```python
from build123d import *

# Parameters (mm, degrees)
SCHIZZO2_R                   = 25.5
TAGLIO_ESTRUSIONE1_DEPTH     = 10
ESTRUSIONE_ESTRUSIONE1_DEPTH = 51
TAGLIO_ESTRUSIONE2_DEPTH     = 51
SCHIZZO6_R                   = 38.5
TAGLIO_ESTRUSIONE3_DEPTH     = 51


with BuildPart() as part:
    # Schizzo1 → Rivoluzione1 (revolve)
    with BuildSketch(Plane.XY):
        Polygon((0, 439), (101.5, 439), (101.5, 0), (76, 0), (76, 413.5), (0, 413.5), align=None)
    revolve(axis=Axis((0, -167.269578169, 0), (0, 1, 0)))

    # Schizzo2 → Taglio-Estrusione1 (cut)
    with BuildSketch(Plane(origin=(0, 439, 0), x_dir=(1, 0, 0), z_dir=(0, 1, 0))):
        Circle(SCHIZZO2_R)
    extrude(amount=-TAGLIO_ESTRUSIONE1_DEPTH, mode=Mode.SUBTRACT)

    # Schizzo4 → Estrusione-Estrusione1 (add)
    with BuildSketch(Plane(origin=(190.786805103, 252.794995721, 165.848439427), x_dir=(0.656059029, 0, -0.75470958), z_dir=(0.533660262, 0.707106781, 0.463903788))):
        with BuildLine():
            Line((-76.603022393, 263.333642433), (-76.603022393, 108.927930028))
            ThreePointArc((-76.603022393, 108.927930028), (0, 32.324907635), (76.603022393, 108.927930028))
            Line((76.603022393, 108.927930028), (76.603022393, 263.333642433))
            Line((76.603022393, 263.333642433), (-76.603022393, 263.333642433))
        make_face()
    estrusione_estrusione1 = extrude(amount=-ESTRUSIONE_ESTRUSIONE1_DEPTH)

    # Schizzo5 → Taglio-Estrusione2 (cut)
    with BuildSketch(Plane(origin=(190.786805103, 252.794995721, 165.848439427), x_dir=(0.845698956, -0.44620463, -0.292736576), z_dir=(0.533660262, 0.707106781, 0.463903788))):
        with BuildLine():
            Line((-9.31111849, 132.840581346), (-106.745545148, 252.622284978))
            Line((-106.745545148, 252.622284978), (-225.596595186, 155.944882946))
            Line((-225.596595186, 155.944882946), (-128.162168528, 36.163179314))
            ThreePointArc((-128.162168528, 36.163179314), (-20.397942493, 25.076355311), (-9.31111849, 132.840581346))
        make_face()
    taglio_estrusione2 = extrude(amount=TAGLIO_ESTRUSIONE2_DEPTH, mode=Mode.SUBTRACT)

    # Schizzo6 → Taglio-Estrusione3 (cut)
    with BuildSketch(Plane(origin=(190.786805103, 252.794995721, 165.848439427), x_dir=(0.845698956, -0.44620463, -0.292736576), z_dir=(0.533660262, 0.707106781, 0.463903788))):
        with Locations((-68.736643509, 84.50188033)):
            Circle(SCHIZZO6_R)
    taglio_estrusione3 = extrude(amount=-TAGLIO_ESTRUSIONE3_DEPTH, mode=Mode.SUBTRACT)

    # Specchia1: Estrusione-Estrusione1, Taglio-Estrusione2, Taglio-Estrusione3 across plane
    add(estrusione_estrusione1.mirror(Plane(origin=(0, 0, 0), x_dir=(0, 0, 1), z_dir=(1, 0, 0))))
    add(taglio_estrusione2.mirror(Plane(origin=(0, 0, 0), x_dir=(0, 0, 1), z_dir=(1, 0, 0))), mode=Mode.SUBTRACT)
    add(taglio_estrusione3.mirror(Plane(origin=(0, 0, 0), x_dir=(0, 0, 1), z_dir=(1, 0, 0))), mode=Mode.SUBTRACT)


solid = part.part
```
Here's how the part is built. I have some questions about the finished solid (model axes, mm). A direction names the side the tool comes from. Round coordinates to 2 decimals unless told otherwise and drop trailing zeros. Loops run counter-clockwise (first coordinate to the right, second up) from the corner with the lowest first, then second, coordinate; pieces in that order, holes last. Notation, with made-up numbers: (15.5, 50.5) -> (34.5, 50.5) arc R11 ccw to (34.5, 56.5) -> close; hole circle Ø11 at (60, 47). An arc over 180 degrees is marked (long way). Answer as CSV lines item,"result". Start each with the question number.
1. Imagine slicing it at C-C on x = -7.5. Write out the boundary of the cut face in (y, z), plus the area to 3 significant figures.
2. If we mould it in two halves opening along X, with no side actions, what happens to faces 4 (the face through (96.63, 376.62, 85.42)), 5 (the face through (-21, 439, -24)), 6 (the face through (-34.94, 408.29, 14.5))? For each: pulls with the +X half, pulls with the -X half, needs draft (parallel to the pull), parting line crosses it, or undercut.
3. For faces 1 (the face through (36.361, 355.264, 133.108)), 2 (the face through (54.566, 216.427, -85.585)), 3 (the face through (34.94, 408.29, 14.5)), which set-ups out of +Z, -Z, +X, -X, +Y, -Y let a thin tool reach every point of the face, with its end or its side?
4. Imagine slicing it at B-B on z = 0. Write out the boundary of the cut face in (x, y), plus the area to 3 significant figures.
5. I'm going to push flat-ended pins straight in: P1, Ø10, axis at x = 2, y = 201, coming from the +Z side; P2, Ø3, axis at y = 206, z = -20.5, coming from the +X side; P3, Ø1, axis at x = -9.5, y = 93, coming from the -Z side. Where does each tip first touch, or does it pass through?
6. Imagine slicing it at A-A on y = 37. Write out the boundary of the cut face in (x, z), plus the area to 3 significant figures.
7. I need wall thicknesses on probe 1 along X at (y, z) = (313, 102); probe 2 along X at (y, z) = (124, 0); probe 3 along Z at (x, y) = (-56.5, 173). Which ranges of each line are inside material? Lowest first, please. Write a range as from..to.
8. Imagine slicing it at D-D on z = 117.5. State how many separate pieces and enclosed holes the cut face has, plus the area to 3 significant figures.
Solution:
1,outline,"(0, -101.22) -> (439, -101.22) -> (439, -24.37) -> (429, -24.37) -> (429, 24.37) -> (439, 24.37) -> (439, 92.87) -> (429.06, 108.02) -> (356.94, 108.02) -> (361.4, 101.22) -> (0, 101.22) -> (0, 75.63) -> (378.19, 75.63) -> (402.94, 37.9) -> (413.5, 54) -> (413.5, -75.63) -> (0, -75.63) -> close"
1,area,"27,100 mm²"
2,face 4,"pulls with the +X half"
2,face 5,"needs draft"
2,face 6,"undercut"
3,face 1,"+Z, +Y, -Y"
3,face 2,"-Y"
3,face 3,"none"
4,outline,"(-116.76, 345.34) -> (-101.5, 356.86) -> (-101.5, 0) -> (-76, 0) -> (-76, 376.11) -> (-40.45, 402.94) -> (-54.44, 413.5) -> (54.44, 413.5) -> (40.45, 402.94) -> (76, 376.11) -> (76, 0) -> (101.5, 0) -> (101.5, 356.86) -> (116.76, 345.34) -> (116.76, 417.47) -> (88.23, 439) -> (25.5, 439) -> (25.5, 429) -> (-25.5, 429) -> (-25.5, 439) -> (-88.23, 439) -> (-116.76, 417.47) -> close"
4,area,"29,400 mm²"
5,P1,"z = 101.5"
5,P2,"x = 99.71"
5,P3,"z = -101.1"
6,outline,"circle Ø203 at (0, 0); hole circle Ø152 at (0, 0)"
6,area,"14,200 mm²"
7,probe 1,"-166.52..-164.64, -73.7..-70.95, 70.95..73.7, 164.64..166.52"
7,probe 2,"-101.5..-76, 76..101.5"
7,probe 3,"-84.32..-50.83, 50.83..84.32"
8,separate pieces,"4"
8,enclosed holes,"0"
8,area,"14,600 mm²"
